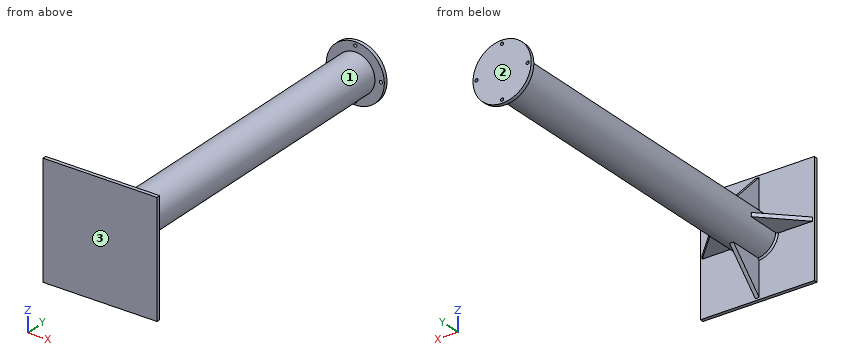
from build123d import *

# Parameters (mm, degrees)
CROQUIS1_R              = 50.8
SALIENTE_EXTRUIR1_DEPTH = 448
CROQUIS2_W              = 294
CROQUIS2_H              = 294
SALIENTE_EXTRUIR2_DEPTH = 9.5
CROQUIS3_R              = 75
SALIENTE_EXTRUIR3_DEPTH = 9.5
CORTAR_EXTRUIR1_REACH   = 940.319
CROQUIS4_R              = 4
MATRIZC1_COUNT          = 4
CHAFL_N1_SIZE           = 4
NERVIO2_REACH           = 504.518
CROQUIS5_WALL_W         = 1136.012097146
CROQUIS5_WALL_H         = 10
MATRIZC2_COUNT          = 4


with BuildPart() as part:
    # Croquis1 → Saliente-Extruir1 (new, symmetric)
    with BuildSketch(Plane(origin=(0, 0, 0), x_dir=(1, 0, 0), z_dir=(0, 1, 0))):
        with Locations(Location((0, 0, 0), (0, 0, 270))):
            Circle(CROQUIS1_R)
    extrude(amount=SALIENTE_EXTRUIR1_DEPTH, both=True)

    # Croquis2 → Saliente-Extruir2 (add)
    with BuildSketch(Plane.XZ.offset(448)):
        Rectangle(CROQUIS2_W, CROQUIS2_H)
    extrude(amount=SALIENTE_EXTRUIR2_DEPTH)

    # Croquis3 → Saliente-Extruir3 (add)
    with BuildSketch(Plane(origin=(0, 448, 0), x_dir=(1, 0, 0), z_dir=(0, 1, 0))):
        with Locations(Location((0, 0, 0), (0, 0, 270))):
            Circle(CROQUIS3_R)
    extrude(amount=SALIENTE_EXTRUIR3_DEPTH)

    # Croquis4 → Cortar-Extruir1 (cut, up to next)
    with BuildSketch(Plane(origin=(0, 457.5, 0), x_dir=(1, 0, 0), z_dir=(0, 1, 0)), mode=Mode.PRIVATE) as cortar_extruir1_sk1:
        with Locations(Location((0, 66, 0), (0, 0, 270))):
            Circle(CROQUIS4_R)
    cortar_extruir1_tool1 = extrude(cortar_extruir1_sk1.sketch, amount=-CORTAR_EXTRUIR1_REACH, mode=Mode.PRIVATE) & part.part
    cortar_extruir1 = cortar_extruir1_tool1.solids().sort_by_distance((0, 457.5, -66))[0]
    add(cortar_extruir1, mode=Mode.SUBTRACT)

    # MatrizC1: Cortar-Extruir1 ×4 about axis
    matrizc1_axis = Axis((0, 0, 0), (0, 1, 0))
    for i in range(1, MATRIZC1_COUNT):
        add(cortar_extruir1.rotate(matrizc1_axis, i * 360 / MATRIZC1_COUNT), mode=Mode.SUBTRACT)

    # Chaflán1
    chafl_n1_edges = [part.edges().sort_by_distance(p)[0] for p in [
        (0, -448, -50.8),
    ]]
    chamfer(chafl_n1_edges, length=CHAFL_N1_SIZE)

    # Croquis5 wall → Nervio2 (add, up to next)
    with BuildSketch(Plane(origin=(-96.4, -402.4, 0), x_dir=(0.707106781187, 0.707106781187, 0), z_dir=(-0.707106781187, 0.707106781187, 0)), mode=Mode.PRIVATE) as nervio2_sk1:
        Rectangle(CROQUIS5_WALL_W, CROQUIS5_WALL_H)
    nervio2_tool1 = extrude(nervio2_sk1.sketch, amount=-NERVIO2_REACH, mode=Mode.PRIVATE) - part.part
    nervio2 = nervio2_tool1.solids().sort_by_distance((-96.4, -402.4, 0))[0]
    add(nervio2)

    # MatrizC2: Nervio2 ×4 about axis
    matrizc2_axis = Axis((0, 0, 0), (0, 1, 0))
    for i in range(1, MATRIZC2_COUNT):
        add(nervio2.rotate(matrizc2_axis, i * 360 / MATRIZC2_COUNT))


solid = part.part
The listing builds one solid part. Answer for the finished solid, in the listing's coordinates (mm). Face numbers are marked on the shaded views. Round coordinates to 2 decimals unless told otherwise and drop trailing zeros. Order: outer loops, then holes, each group sorted by start corner. A loop starts at its lowest first (then second) coordinate and runs counter-clockwise, first axis right, second up. Notation, with made-up numbers: (65, -13.75) -> (83, -13.75) arc R4 cw to (83, -8.75) -> close; hole circle Ø4 at (-5.75, 82). An arc over 180 degrees is marked (long way). Put each result on its own line as item: value.
Q1. Consider line 1 along Y through (x, z) = (-107, -81); line 2 along Z through (x, y) = (66, 455). Determine where each line is inside the solid, lowest interval first.
Results list:
line 1: -457.5 to -448
line 2: -35.62 to -4, 4 to 35.62
Q2. Section C-C, the plane z = -107 is taken. Write down the section's boundary in (x, y).
Results list:
outline: (-147, -457.5) -> (147, -457.5) -> (147, -448) -> (5, -448) -> (5, -413) -> (-5, -413) -> (-5, -448) -> (-147, -448) -> close
Q3. Section D-D, the plane y = 288 is taken. Write down the section's boundary in (x, z), and give its area (3 significant figures).
Results list:
outline: circle Ø101.6 at (0, 0)
area: 8,110 mm^2
Q4. Section A-A, the plane x = 86 is taken. Write down the section's boundary in (y, z).
Results list:
outline: (-457.5, -147) -> (-448, -147) -> (-448, -5) -> (-392, -5) -> (-392, 5) -> (-448, 5) -> (-448, 147) -> (-457.5, 147) -> close
Q5. Each of these flat-tipped pins is pushed along its axis until it touches: P1, Ø10, axis at y = 319, z = -18.5, coming from the -X side; P2, Ø4, axis at x = 40.5, y = 33, coming from the -Z side; P3, Ø3, axis at y = 353, z = -43, coming from the +X side. Where does it stop, or does it pass through?
Results list:
P1: x = -48.97
P2: z = -33.14
P3: x = 29.3
Q6. Section B-B, the plane y = -391 is taken. Write down the section's boundary in (x, z), and give its area (3 significant figures).
Results list:
outline: (-85, -5) -> (-50.55, -5) arc R50.8 ccw to (-5, -50.55) -> (-5, -85) -> (5, -85) -> (5, -50.55) arc R50.8 ccw to (50.55, -5) -> (85, -5) -> (85, 5) -> (50.55, 5) arc R50.8 ccw to (5, 50.55) -> (5, 85) -> (-5, 85) -> (-5, 50.55) arc R50.8 ccw to (-50.55, 5) -> (-85, 5) -> close
area: 9,480 mm^2
Q7. Determine the mould class of the marked faces 1, 2 and 3 for opening direction Y: pulls with the +Y half, pulls with the -Y half, needs draft (parallel to the pull), parting line crosses it, or undercut.
Results list:
face 1: undercut
face 2: pulls with the +Y half
face 3: pulls with the -Y half
